Geometry: final body of the model. Coordinates: model frame, mm. A direction names the side the tool comes from. Give positions to 0.01 mm unless a question says otherwise; leave off trailing zeros. Order: outer loops, then holes, each group sorted by start corner. A loop starts at its lowest first (then second) coordinate and runs counter-clockwise, first axis right, second up. Notation, with made-up numbers: (-39.5, -17.5) - (-17.5, -17.5) arc R5 ccw to (-17.5, -9.5) - close; hole circle Ø3 at (66.25, -8). An arc over 180 degrees is marked (long way). One line per item, written item: value.
```python
from build123d import *

# Parameters (mm, degrees)
BOSS_EXTRU_1_DEPTH      = 130
ESQUISSE3_R             = 10
ENL_V_MAT_EXTRU_1_DEPTH = 40
CONG_1_R                = 2
CONG_2_R                = 2


with BuildPart() as part:
    # Esquisse2 → Boss.-Extru.1 (new body)
    with BuildSketch(Plane.XY):
        Polygon((0, 0), (-215.549768864, 0), (-215.549768864, 145.390154902), align=None)
    extrude(amount=BOSS_EXTRU_1_DEPTH)

    # Esquisse3 → Enlèv. mat.-Extru.1 (cut)
    with BuildSketch(Plane(origin=(0, 0, 0), x_dir=(0.829037573, -0.559192903, 0), z_dir=(0.559192903, 0.829037573, 0))):
        with Locations((-120, -19.80283687)):
            Circle(ESQUISSE3_R)
        with Locations((-120, -110.19716313)):
            Circle(ESQUISSE3_R)
    extrude(amount=-ENL_V_MAT_EXTRU_1_DEPTH, mode=Mode.SUBTRACT)

    # Congé1
    cong_1_edges = [part.edges().sort_by_distance(p)[0] for p in [
        (-130.142600571, 39.533574549, 19.80283687),
    ]]
    fillet(cong_1_edges, radius=CONG_1_R)

    # Congé2
    cong_2_edges = [part.edges().sort_by_distance(p)[0] for p in [
        (-130.142600571, 39.533574549, 110.19716313),
    ]]
    fillet(cong_2_edges, radius=CONG_2_R)


solid = part.part
```
1) Mould query, pull axis X, two halves, no side actions, for faces 3 (the face through (-109.28, 73.71, 64.09)), 4 (the face through (-215.55, 72, 64)), 5 (the face through (-154, 41, 0)), 6 (the face through (-116.54, 56.01, 116.28)). Classes: released by +X, released by -X, zero draft, split by the parting line, or undercut.
Answers below:
face 3: released by +X
face 4: released by -X
face 5: zero draft
face 6: undercut
2) First-contact query: pin 1 (1 mm diameter, centred on x = -139.5, z = 18.5, fed in from -Y). Flat tip, straight axial feed; report the tip coordinate or a pass-through.
Answers below:
pin 1: y = 0
3) Section C-C, the plane x = -39. Return loops of the section in (y, z), then the cut area to 3 significant figures.
Answers below:
outline: (0, 0) - (26.31, 0) - (26.31, 130) - (0, 130) - close
area: 3,420 mm^2
4) Set-up query: faces 1 (the face through (-106, 0, 64)), 2 (the face through (-121.945, 34.004, 19.691)). Return all of +Z, -Z, +X, -X, +Y, -Y with unobstructed straight access to the full face (end or side cutting, diameter ignored); none if empty.
Answers below:
face 1: +Z, -Z, +X, -X, -Y
face 2: none
5) Material intervals for line 1 along X through (y, z) = (69, 88); line 2 along X through (y, z) = (59.5, 87.5); line 3 along Y through (x, z) = (-178.5, 74), sorted ascending.
Answers below:
line 1: -215.55 to -102.3
line 2: -215.55 to -88.21
line 3: 0 to 120.4
6) Section D-D, the plane y = 50.5. Count the separate pieces of the cut face and the enclosed holes in it, then the cut area to 3 significant figures.
Answers below:
separate pieces: 1
enclosed holes: 2
area: 17,500 mm^2
7) Section B-B, the plane y = 132.5. Return loops of the section in (x, z), then the cut area to 3 significant figures.
Answers below:
outline: (-215.55, 0) - (-196.44, 0) - (-196.44, 130) - (-215.55, 130) - close
area: 2,480 mm^2
8) Section A-A, the plane z = 70.5. Return loops of the section in (x, y).
Answers below:
outline: (-215.55, 0) - (0, 0) - (-215.55, 145.39) - close
